from build123d import *

# Parameters (mm, degrees)
F1_DEPTH = 1.5875
F3_DEPTH = 1.5875
F4_R     = 0.79375
F5_DEPTH = 25.4


with BuildPart() as f1:
    # F0 (on Top) → F1 (new body)
    with BuildSketch(Plane.XY):
        Polygon((-14.929745, 4.850968), (-9.22709, -12.7), (9.22709, -12.7), (14.929745, 4.850968), (0, 15.698063), align=None)
    extrude(amount=F1_DEPTH)

    # F2 (on face) → F3 (join)
    with BuildSketch(Plane.XY.offset(1.5875)):
        with BuildLine():
            Line((-11.407689, -0.713822), (-12.676007, -0.780292))
            ThreePointArc((-12.676007, -0.780292), (-12.476655, -2.371304), (-12.078418, -3.924516))
            Line((-12.078418, -3.924516), (-10.870576, -3.532064))
            ThreePointArc((-10.870576, -3.532064), (-11.227907, -2.139862), (-11.407689, -0.713822))
        make_face()
        with BuildLine():
            Line((-10.870576, -3.532064), (-12.078418, -3.924516))
            ThreePointArc((-12.078418, -3.924516), (-11.487643, -5.415169), (-10.713749, -6.819501))
            Line((-10.713749, -6.819501), (-9.648588, -6.127777))
            ThreePointArc((-9.648588, -6.127777), (-10.341347, -4.868413), (-10.870576, -3.532064))
        make_face()
        with BuildLine():
            ThreePointArc((-4.659203, 11.814475), (-6.110742, 11.133231), (-7.464873, 10.274516))
            Line((-7.464873, 10.274516), (-6.718385, 9.247064))
            ThreePointArc((-6.718385, 9.247064), (-5.504744, 10.01712), (-4.204055, 10.628773))
            Line((-4.204055, 10.628773), (-4.659203, 11.814475))
        make_face()
        with BuildLine():
            Line((-6.718385, 9.247064), (-7.464873, 10.274516))
            ThreePointArc((-7.464873, 10.274516), (-8.700008, 9.252019), (-9.796461, 8.082039))
            Line((-9.796461, 8.082039), (-8.80944, 7.282765))
            ThreePointArc((-8.80944, 7.282765), (-7.825788, 8.330783), (-6.718385, 9.247064))
        make_face()
        with BuildLine():
            ThreePointArc((-3.175, -12.296722), (-1.600255, -12.598777), (0, -12.7))
            Line((0, -12.7), (0, -11.43))
            ThreePointArc((0, -11.43), (-1.434484, -11.339628), (-2.846285, -11.06994))
            Line((-2.846285, -11.06994), (-3.175, -12.296722))
        make_face()
        with BuildLine():
            Line((0, -11.43), (0, -12.7))
            ThreePointArc((0, -12.7), (1.600255, -12.598777), (3.175, -12.296722))
            Line((3.175, -12.296722), (2.846285, -11.06994))
            ThreePointArc((2.846285, -11.06994), (1.434484, -11.339628), (0, -11.43))
        make_face()
        with BuildLine():
            ThreePointArc((10.713749, -6.819501), (11.487643, -5.415169), (12.078418, -3.924516))
            Line((12.078418, -3.924516), (10.870576, -3.532064))
            ThreePointArc((10.870576, -3.532064), (10.341347, -4.868413), (9.648588, -6.127777))
            Line((9.648588, -6.127777), (10.713749, -6.819501))
        make_face()
        with BuildLine():
            Line((10.870576, -3.532064), (12.078418, -3.924516))
            ThreePointArc((12.078418, -3.924516), (12.476655, -2.371304), (12.676007, -0.780292))
            Line((12.676007, -0.780292), (11.407689, -0.713822))
            ThreePointArc((11.407689, -0.713822), (11.227907, -2.139862), (10.870576, -3.532064))
        make_face()
        with BuildLine():
            ThreePointArc((9.796461, 8.082039), (8.700008, 9.252019), (7.464873, 10.274516))
            Line((7.464873, 10.274516), (6.718385, 9.247064))
            ThreePointArc((6.718385, 9.247064), (7.825788, 8.330783), (8.80944, 7.282765))
            Line((8.80944, 7.282765), (9.796461, 8.082039))
        make_face()
        with BuildLine():
            Line((6.718385, 9.247064), (7.464873, 10.274516))
            ThreePointArc((7.464873, 10.274516), (6.110742, 11.133231), (4.659203, 11.814475))
            Line((4.659203, 11.814475), (4.204055, 10.628773))
            ThreePointArc((4.204055, 10.628773), (5.504744, 10.01712), (6.718385, 9.247064))
        make_face()
        Polygon((8.248892, 4.7625), (-8.248892, 4.7625), (0, -9.525), align=None)
    extrude(amount=F3_DEPTH)

    # F4 (on face) → F5 (cut)
    with BuildSketch(Plane.XY.offset(1.5875)):
        with Locations((0, 13.49375)):
            Circle(F4_R)
    extrude(amount=-F5_DEPTH, mode=Mode.SUBTRACT)


solid = f1.part
Can you work these out from the model? Positions are in its coordinate system, mm. A direction names the side the tool comes from. Coordinates: 2 decimals unless noted, no trailing zeros. Order: outer loops, then holes, each group sorted by start corner. A loop starts at its lowest first (then second) coordinate and runs counter-clockwise, first axis right, second up. Notation, with made-up numbers: (87.5, 88) -> (93.5, 88) arc R22 cw to (93.5, 107) -> close; hole circle Ø8 at (27.5, -24). An arc over 180 degrees is marked (long way). Use one line per item in the form item = value.
Q1. Imagine slicing it at A-A, the plane y = 3.75. List the corners of the cut face in (x, z) for me (1 decimal).
From the geometry:
outline = (-14.6, 0) -> (14.6, 0) -> (14.6, 1.6) -> (7.7, 1.6) -> (7.7, 3.2) -> (-7.7, 3.2) -> (-7.7, 1.6) -> (-14.6, 1.6) -> close
Q2. Which directions (+Z, -Z, +X, -X, +Y, -Y) give clear straight access to the entire face, cutting with the end or side of a thin tool? Please do faces 1 (the face through (-4.182, -2.281, 2.37)), 2 (the face through (-12.48, -2.35, 2.37)), 3 (the face through (-12.033, -0.747, 2.37)).
From the geometry:
face_1 = +Z
face_2 = +Z, -X, -Y
face_3 = +Z, -X, +Y
Q3. Will these pins go through, and if not, where does the flat tip stop? P1, Ø1.5, axis at y = -6.5, z = 2.5, coming from the +X side; P2, Ø0.5, axis at x = 1, z = 2, coming from the +Y side.
From the geometry:
P1 = 11.32
P2 = 4.76
Q4. We'd pull the mould along Y, two halves only. Please class faces 4 (the face through (0, 4.762, 2)), 5 (the face through (0, -12, 3.175)), 6 (the face through (-3.008, -11.675, 2.37)), 7 (the face through (8.716, 9.237, 2.37)): released by +Y, released by -Y, zero draft, split by the parting line, or undercut.
From the geometry:
face_4 = undercut
face_5 = zero draft
face_6 = undercut
face_7 = released by +Y
Q5. I need wall thicknesses on L1, parallel to Z at x = 4.75, y = 9; L2, parallel to X at y = 11.5, z = 2.7; L3, parallel to X at y = -6, z = 1.85. Which ranges of each line are inside material? Lowest first, please.
From the geometry:
L1 = 0 to 1.59
L2 = -5.39 to -4.54, 4.54 to 5.39
L3 = -11.19 to -9.73, -2.04 to 2.04, 9.73 to 11.19
Q6. Imagine slicing it at C-C, the plane y = 8.5. List the corners of the cut face in (x, z) for me (1 decimal).
From the geometry:
outline = (-9.9, 0) -> (9.9, 0) -> (9.9, 1.6) -> (9.4, 1.6) -> (9.4, 3.2) -> (7.6, 3.2) -> (7.6, 1.6) -> (-7.6, 1.6) -> (-7.6, 3.2) -> (-9.4, 3.2) -> (-9.4, 1.6) -> (-9.9, 1.6) -> close
